Here's how the part is built. I have some questions about the finished solid (model axes, mm). Face numbers are marked on the shaded views. A direction names the side the tool comes from. Coordinates: 2 decimals unless noted, no trailing zeros. Write each loop counter-clockwise with the first axis right and the second up, starting at its lowest first coordinate (ties: lowest second). Pieces come first, ordered by that corner, then holes. Notation, with made-up numbers: (36.25, -28.5) -> (81.25, -28.5) arc R25 ccw to (81.25, -2.5) -> close; hole circle Ø1 at (15.5, -16.5). An arc over 180 degrees is marked (long way). Use a Markdown table: item, result. Add a question column.
Item 1: Imagine slicing it at C-C, the plane y = 4.25. Write out the boundary of the cut face in (x, z).
Item 2: Imagine slicing it at A-A, the plane x = 0. Write out the boundary of the cut face in (y, z), and give its area (4 significant figures).
Item 3: If we mould it in two halves opening along X, with no side actions, what happens to the marked faces 1, 2 and 3? For each: pulls with the +X half, pulls with the -X half, needs draft (parallel to the pull), parting line crosses it, or undercut.
Item 4: Imagine slicing it at B-B, the plane y = -4.5. Write out the boundary of the cut face in (x, z).
Item 5: If I drill on line 1 along Z through (x, y) = (0, -9); line 2 along X through (y, z) = (-10, -10); line 3 along Z through (x, y) = (-3.5, -3), over which ranges is the centre line in solid material (lowest first)? Write a range as from..to.
Item 6: On a 3-axis mill with a long thin cutter (end or side, diameter ignored), from which of +Z, -Z, +X, -X, +Y, -Y can I reach the whole of each face in a straight line? I mean the marked faces 4, 5, 6 and 7. Say none if no direction works.
Item 7: Will these pins go through, and if not, where does the flat tip stop? pin 1 Ø1.5 at (x, y) = (8.5, -9.5) entering from -Z; pin 2 Ø5 at (y, z) = (2.5, -16) entering from +X; pin 3 Ø7 at (x, z) = (0, -10) entering from -Y; pin 4 Ø6 at (x, y) = (6.5, -9.5) entering from -Z.
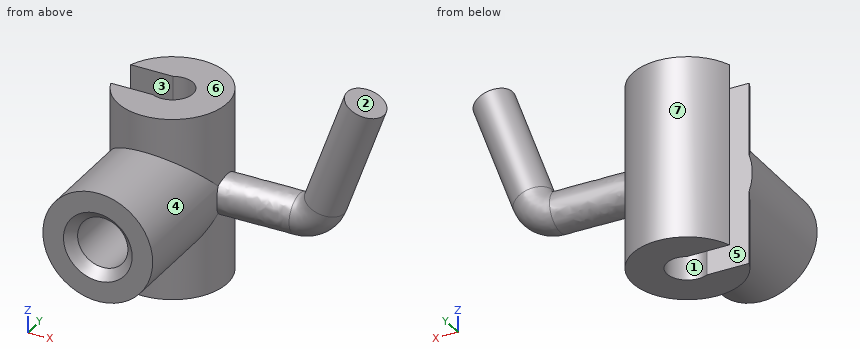
```python
from build123d import *

# Parameters (mm, degrees)
F0_R      = 6
F1_DEPTH  = 20
F4_R      = 6
F4_R_2    = 2.75
F5_DEPTH  = 15
F7_DEPTH  = 20
F8_SIZE   = 1
F11_R     = 2.15
F2_R      = 2.25
F13_DEPTH = 20.0010001


# Not quite as in the source:
# - a feature of the source that left no trace in its solid (it failed there, or was rolled back) is left out


with BuildPart() as f1:
    # F0 (on Top) → F1 (new body)
    with BuildSketch(Plane.XY):
        Circle(F0_R)
    extrude(amount=-F1_DEPTH)

    # F4 (on offset) → F5 (join)
    with BuildSketch(Plane.XZ.offset(15)):
        with Locations((0, -10)):
            Circle(F4_R)
        with Locations((0, -10)):
            Circle(F4_R_2, mode=Mode.SUBTRACT)
    extrude(amount=-F5_DEPTH)

    # F6 (on face) → F7 (cut, through all)
    with BuildSketch(Plane.XY):
        with BuildLine():
            Line((0, 2), (-5.6568542495, 2))
            ThreePointArc((-5.6568542495, 2), (-6, 0), (-5.6568542495, -2))
            Line((-5.6568542495, -2), (0, -2))
            Line((0, -2), (0, 2))
        make_face()
        with BuildLine():
            Line((-5.6568542495, 2), (-8.5344118631, 2))
            Line((-8.5344118631, 2), (-8.5344118631, -2))
            Line((-8.5344118631, -2), (-5.6568542495, -2))
            ThreePointArc((-5.6568542495, -2), (-6, 0), (-5.6568542495, 2))
        make_face()
    extrude(amount=-F7_DEPTH, mode=Mode.SUBTRACT)

    # F8
    f8_edges = [f1.edges().sort_by_distance(p)[0] for p in [
        (-2.75, -15, -10),
    ]]
    chamfer(f8_edges, length=F8_SIZE)

    # F12: sweep along a path in F10
    with BuildLine(Plane.XZ) as f12_path:
        Line((0, -10), (13.8992802655, -9.9480403702))
        ThreePointArc((13.8992802655, -9.9480403702), (15.6179693755, -9.3990677428), (16.7109593102, -7.9635761178))
        Line((16.7109593102, -7.9635761178), (21.0774621296, 4.1742816034))
    # F11 (on offset) → F12 (sweep)
    with BuildSketch(Plane.YZ.offset(6)):
        with Locations((0, -10)):
            Circle(F11_R)
    sweep(path=f12_path.line)

    # F2 (on face) → F13 (cut, through all)
    with BuildSketch(Plane.XY):
        Circle(F2_R)
    extrude(amount=-F13_DEPTH, mode=Mode.SUBTRACT)


solid = f1.part
```
Ans:
| question | item | result |
|---|---|---|
| 1 | outline | (-4.24, -20) -> (4.24, -20) -> (4.24, 0) -> (-4.24, 0) -> close |
| 2 | outline | (-15, -16) -> (-6, -16) -> (-6, -20) -> (-2.25, -20) -> (-2.25, 0) -> (-6, 0) -> (-6, -4) -> (-15, -4) -> (-15, -6.25) -> (-14, -7.25) -> (-6, -7.25) -> (-6, -12.75) -> (-14, -12.75) -> (-15, -13.75) -> close; (2.25, -20) -> (6, -20) -> (6, 0) -> (2.25, 0) -> close |
| 2 | area | 207.5 mm^2 |
| 3 | face 1 | undercut |
| 3 | face 2 | pulls with the +X half |
| 3 | face 3 | needs draft |
| 4 | outline | (-3.97, -20) -> (3.97, -20) -> (3.97, -14.5) arc R6 ccw to (3.97, -5.5) -> (3.97, 0) -> (-3.97, 0) -> (-3.97, -5.5) arc R6 ccw to (-3.97, -14.5) -> close |
| 5 | line 1 | z = -16..-12.75, -7.25..-4 |
| 5 | line 2 | x = -6..-2.75, 2.75..6 |
| 5 | line 3 | z = -20..0 |
| 6 | face 4 | -Y |
| 6 | face 5 | +Z, -Z, -X |
| 6 | face 6 | +Z, -X, +Y, -Y |
| 6 | face 7 | none |
| 7 | pin 1 | passes through |
| 7 | pin 2 | stops at x = 6 |
| 7 | pin 3 | stops at y = -14.75 |
| 7 | pin 4 | stops at z = -14.87 |
